Input: part model. Units: mm. Frame: model coordinates. Face numbers are marked on the shaded views. A direction names the side the tool comes from. Coordinates: 2 decimals unless noted, no trailing zeros. Order: outer loops, then holes, each group sorted by start corner. A loop starts at its lowest first (then second) coordinate and runs counter-clockwise, first axis right, second up. Notation, with made-up numbers: (45, 45.25) -> (79, 45.25) arc R36 ccw to (79, 84.25) -> close; hole circle Ø5 at (25, 47.5). An arc over 180 degrees is marked (long way). Write each question's results on one line, items separated by ' | '.
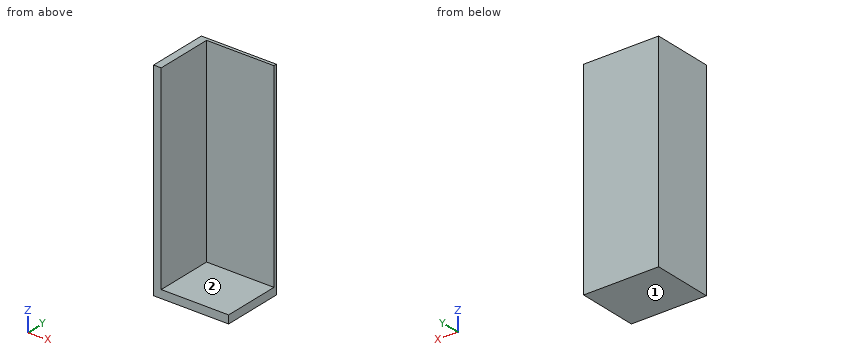
```python
from build123d import *

# Parameters (mm, degrees)
SKETCH1_R           = 28.1
BOSS_EXTRUDE1_DEPTH = 1
SKETCH2_R           = 18.6
CUT_EXTRUDE1_DEPTH  = 58.8
SKETCH3_W           = 222.683092022
SKETCH3_H           = 364.2827524
BOSS_EXTRUDE2_DEPTH = 58.8
SKETCH4_W           = 207.917403516
SKETCH4_H           = 348.54429772
CUT_EXTRUDE2_DEPTH  = 55.8
SKETCH9_R           = 3
CUT_EXTRUDE8_DEPTH  = 10
SKETCH10_R          = 3.75
CUT_EXTRUDE9_DEPTH  = 10
CUT_EXTRUDE12_DEPTH = 500
SKETCH6_R           = 3.75
CUT_EXTRUDE5_DEPTH  = 400
SKETCH8_R           = 10
CUT_EXTRUDE7_DEPTH  = 10


with BuildPart() as part:
    # Sketch1 → Boss-Extrude1 (new body)
    with BuildSketch(Plane(origin=(0, 0, 0), x_dir=(1, 0, 0), z_dir=(0, 1, 0))):
        Circle(SKETCH1_R)
    extrude(amount=BOSS_EXTRUDE1_DEPTH)

    # Sketch2 → Cut-Extrude1 (cut)
    with BuildSketch(Plane(origin=(0, 1, 0), x_dir=(1, 0, 0), z_dir=(0, 1, 0))):
        with Locations((0, -7)):
            Circle(SKETCH2_R)
    extrude(amount=-CUT_EXTRUDE1_DEPTH, mode=Mode.SUBTRACT)

    # Sketch3 → Boss-Extrude2 (add)
    with BuildSketch(Plane(origin=(0, 0, 0), x_dir=(-1, 0, 0), z_dir=(0, -1, 0))):
        Rectangle(SKETCH3_W, SKETCH3_H)
    extrude(amount=BOSS_EXTRUDE2_DEPTH)

    # Sketch4 → Cut-Extrude2 (cut)
    with BuildSketch(Plane(origin=(0, -58.8, 0), x_dir=(-1, 0, 0), z_dir=(0, -1, 0))):
        Rectangle(SKETCH4_W, SKETCH4_H)
    extrude(amount=-CUT_EXTRUDE2_DEPTH, mode=Mode.SUBTRACT)

    # Sketch9 → Cut-Extrude8 (cut)
    with BuildSketch(Plane(origin=(0, 0, 0), x_dir=(1, 0, 0), z_dir=(0, 1, 0))):
        with Locations((0, -7)):
            Circle(SKETCH9_R)
    extrude(amount=-CUT_EXTRUDE8_DEPTH, mode=Mode.SUBTRACT)

    # Sketch10 → Cut-Extrude9 (cut)
    with BuildSketch(Plane(origin=(0, 1, 0), x_dir=(1, 0, 0), z_dir=(0, 1, 0))):
        with Locations((0, 19.85)):
            Circle(SKETCH10_R)
    extrude(amount=-CUT_EXTRUDE9_DEPTH, mode=Mode.SUBTRACT)

    # Sketch11 → Cut-Extrude12 (cut)
    with BuildSketch(Plane(origin=(0, -58.8, 0), x_dir=(-1, 0, 0), z_dir=(0, -1, 0))):
        Polygon((38.658453989, -17.8586238), (111.341546011, -17.8586238), (111.341546011, -182.1413762), (-111.341546011, -182.1413762), (-111.341546011, 182.1413762), (38.658453989, 182.1413762), align=None)
    extrude(amount=-CUT_EXTRUDE12_DEPTH, mode=Mode.SUBTRACT)

    # Sketch6 → Cut-Extrude5 (cut)
    with BuildSketch(Plane(origin=(0, 1, 0), x_dir=(1, 0, 0), z_dir=(0, 1, 0))):
        with Locations((0, 18.75)):
            Circle(SKETCH6_R)
    extrude(amount=-CUT_EXTRUDE5_DEPTH, mode=Mode.SUBTRACT)

    # Sketch8 → Cut-Extrude7 (cut)
    with BuildSketch(Plane(origin=(0, 0, -182.1413762), x_dir=(-1, 0, 0), z_dir=(0, 0, -1))):
        with Locations((-86.573671766, -25.011155335)):
            Circle(SKETCH8_R)
    extrude(amount=-CUT_EXTRUDE7_DEPTH, mode=Mode.SUBTRACT)


solid = part.part
```
(1) Reachability of the marked faces 1 and 2 from +Z, -Z, +X, -X, +Y, -Y: full face, straight path, thin tool, end or side. Return the list, or none.
Return value:
face 1: -Z, +X, -X, +Y, -Y | face 2: +Z, +X, -Y
(2) Cut plane A-A, the plane x = -52.5. Return loops of the section in (y, z).
Return value:
outline: (-58.8, -182.14) -> (0, -182.14) -> (0, 17.86) -> (-3, 17.86) -> (-3, -174.27) -> (-58.8, -174.27) -> close
(3) Line query: line 1 along X through (y, z) = (-39.5, -87.5); line 2 along Z through (x, y) = (-50.5, -39); line 3 along Y through (x, z) = (-43.5, -141.5). Output: solid intervals per line, ascending. Write a range as from..to.
Return value:
line 1: -111.34..-103.96 | line 2: -182.14..-174.27 | line 3: -3..0
(4) Pin query (flat end, axial travel): P1, Ø4, axis at y = -37.5, z = -94, coming from the +X side; P2, Ø16.5, axis at x = -72, y = -23.5, coming from the +Z side; P3, Ø8, axis at x = -80.5, z = -100.5, coming from the -Y side. Return the tip coordinate at first contact, or that it passes through.
Return value:
P1: x = -103.96 | P2: z = -174.27 | P3: y = -3
(5) Cut plane B-B, the plane y = -22. Return loops of the section in (x, z), plus the area to 3 significant figures.
Return value:
outline: (-111.34, -182.14) -> (-38.66, -182.14) -> (-38.66, -174.27) -> (-103.96, -174.27) -> (-103.96, 17.86) -> (-111.34, 17.86) -> close | area: 1,990 mm2
